Part model, mm, in its own coordinate system. Round coordinates to 2 decimals unless told otherwise and drop trailing zeros. Loops run counter-clockwise (first coordinate to the right, second up) from the corner with the lowest first, then second, coordinate; pieces in that order, holes last. Notation, with made-up numbers: (-36.5, -17.75) -> (-19.5, -17.75) arc R18 ccw to (-19.5, 1.25) -> close; hole circle Ø4 at (13.25, -3). An arc over 180 degrees is marked (long way). Answer as CSV lines item,"result".
from build123d import *

# Parameters (mm, degrees)
ESQUISSE1_W             = 780
ESQUISSE1_H             = 30
BASE_EXTRUSION_DEPTH    = 30
ESQUISSE3_R             = 15
ENL_V_MAT_EXTRU_1_DEPTH = 702.284535691


with BuildPart() as part:
    # Esquisse1 → Base-Extrusion (new, symmetric)
    with BuildSketch(Plane.XY):
        with Locations((-310, -375)):
            Rectangle(ESQUISSE1_W, ESQUISSE1_H)
    extrude(amount=BASE_EXTRUSION_DEPTH, both=True)

    # Esquisse3 → Enlèv. mat.-Extru.1 (cut, through all)
    with BuildSketch(Plane(origin=(0, -360, 0), x_dir=(-1, 0, 0), z_dir=(0, 1, 0))):
        with Locations(Location((-60, 0, 0), (0, 0, 90))):
            Circle(ESQUISSE3_R)
    extrude(amount=-ENL_V_MAT_EXTRU_1_DEPTH, mode=Mode.SUBTRACT)


solid = part.part
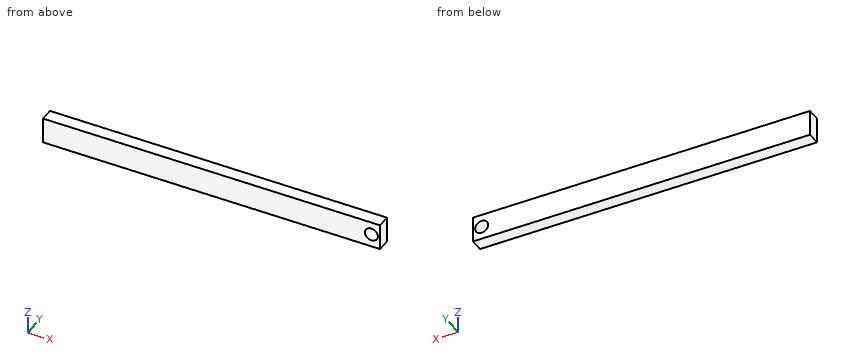
Q1. Saw through at B-B, the plane x = 60. Write the cut outline in (y, z), then the cut area to 3 significant figures.
Geometry results:
outline,"(-390, -30) -> (-360, -30) -> (-360, -15) -> (-390, -15) -> close; (-390, 15) -> (-360, 15) -> (-360, 30) -> (-390, 30) -> close"
area,"900 mm2"
Q2. Saw through at A-A, the plane z = 0. Write the cut outline in (x, y), then the cut area to 3 significant figures.
Geometry results:
outline,"(-700, -390) -> (45, -390) -> (45, -360) -> (-700, -360) -> close; (75, -390) -> (80, -390) -> (80, -360) -> (75, -360) -> close"
area,"22,500 mm2"
Q3. Drill centre line: line 1 along X through (y, z) = (-369.25, 0). Where is it in solid material? Low to high.
Geometry results:
line 1,"-700 to 45, 75 to 80"
